from build123d import *

# Parameters (mm, degrees)
SKETCH1_W           = 65.4
SKETCH1_H           = 65.4
BOSS_EXTRUDE1_DEPTH = 1.12
FILLET1_R           = 4
BOSS_EXTRUDE2_START = 10
BOSS_EXTRUDE2_DEPTH = 10
CUT_EXTRUDE1_REACH  = 75.96
SKETCH4_W           = 19.5
SKETCH4_H           = 3.5
CUT_EXTRUDE2_DEPTH  = 2.5
FILLET3_R           = 2
SKETCH5_W           = 1.6
SKETCH5_H           = 49.8
SKETCH5_W_2         = 49.8
SKETCH5_H_2         = 1.6
BOSS_EXTRUDE3_DEPTH = 1
BOSS_EXTRUDE4_DEPTH = 3.8
SKETCH7_R           = 1.55
CUT_EXTRUDE3_DEPTH  = 11.12
SKETCH8_R           = 2.75
CUT_EXTRUDE4_DEPTH  = 4
FILLET4_R           = 1.5
FILLET5_R           = 1.5
CUT_EXTRUDE5_REACH  = 49.807


with BuildPart() as part:
    # Sketch1 → Boss-Extrude1 (new body)
    with BuildSketch(Plane(origin=(0, 0, 0), x_dir=(1, 0, 0), z_dir=(0, 1, 0))):
        Rectangle(SKETCH1_W, SKETCH1_H)
    extrude(amount=BOSS_EXTRUDE1_DEPTH)

    # Fillet1
    fillet1_edges = [part.edges().sort_by_distance(p)[0] for p in [
        (32.7, 0.56, 32.7),
        (-32.7, 0.56, 32.7),
        (-32.7, 0.56, -32.7),
        (32.7, 0.56, -32.7),
    ]]
    fillet(fillet1_edges, radius=FILLET1_R)

    # Sketch2 → Boss-Extrude2 (add)
    with BuildSketch(Plane(origin=(0, 1.12, 0), x_dir=(1, 0, 0), z_dir=(0, 1, 0)).offset(BOSS_EXTRUDE2_START)):
        with BuildLine():
            Line((-32.7, 28.7), (-32.7, -28.7))
            ThreePointArc((-32.7, -28.7), (-31.528427125, -31.528427125), (-28.7, -32.7))
            Line((-28.7, -32.7), (28.7, -32.7))
            ThreePointArc((28.7, -32.7), (31.528427125, -31.528427125), (32.7, -28.7))
            Line((32.7, -28.7), (32.7, 28.7))
            ThreePointArc((32.7, 28.7), (31.528427125, 31.528427125), (28.7, 32.7))
            Line((28.7, 32.7), (-28.7, 32.7))
            ThreePointArc((-28.7, 32.7), (-31.528427125, 31.528427125), (-32.7, 28.7))
        make_face()
        with BuildLine():
            Line((24.9, 28.7), (-24.9, 28.7))
            ThreePointArc((-24.9, 28.7), (-26.012994231, 26.012994231), (-28.7, 24.9))
            Line((-28.7, 24.9), (-28.7, -24.9))
            ThreePointArc((-28.7, -24.9), (-26.012994231, -26.012994231), (-24.9, -28.7))
            Line((-24.9, -28.7), (24.9, -28.7))
            ThreePointArc((24.9, -28.7), (26.012994231, -26.012994231), (28.7, -24.9))
            Line((28.7, -24.9), (28.7, 24.9))
            ThreePointArc((28.7, 24.9), (26.012994231, 26.012994231), (24.9, 28.7))
        make_face(mode=Mode.SUBTRACT)
    extrude(amount=-BOSS_EXTRUDE2_DEPTH)

    # Sketch3 → Cut-Extrude1 (cut, up to next)
    with BuildSketch(Plane(origin=(0, 0, -32.7), x_dir=(-1, 0, 0), z_dir=(0, 0, -1)), mode=Mode.PRIVATE) as cut_extrude1_sk1:
        with BuildLine():
            Line((-3, 6.5), (3, 6.5))
            ThreePointArc((3, 6.5), (5, 4.5), (3, 2.5))
            Line((3, 2.5), (-3, 2.5))
            ThreePointArc((-3, 2.5), (-5, 4.5), (-3, 6.5))
        make_face()
    cut_extrude1_tool1 = extrude(cut_extrude1_sk1.sketch, amount=-CUT_EXTRUDE1_REACH, mode=Mode.PRIVATE) & part.part
    add(cut_extrude1_tool1.solids().sort_by_distance((0, 4.5, -32.7))[0], mode=Mode.SUBTRACT)

    # Sketch4 → Cut-Extrude2 (cut)
    with BuildSketch(Plane.XY.offset(-28.7)):
        with Locations((0, 2.87)):
            Rectangle(SKETCH4_W, SKETCH4_H)
    extrude(amount=-CUT_EXTRUDE2_DEPTH, mode=Mode.SUBTRACT)

    # Fillet3
    # the kernel refuses this fillet: 2 mm, written as the material it takes off along each edge
    with BuildSketch(Plane(origin=(-0.003603246, 4.62, -28.7), x_dir=(0, 1, 0), z_dir=(1, 0, 0)), Plane(origin=(-9.75, 4.62, -28.7), x_dir=(0, 1, 0), z_dir=(1, 0, 0))) as fillet3_piece_1:
        with BuildLine():
            CenterArc((FILLET3_R, -FILLET3_R), FILLET3_R, 90, 90)
            Line((0, -FILLET3_R), (0, 0))
            Line((0, 0), (FILLET3_R, 0))
        make_face()
    extrude(amount=9.753603246, mode=Mode.SUBTRACT)

    # Sketch5 → Boss-Extrude3 (add)
    with BuildSketch(Plane(origin=(0, 11.12, 0), x_dir=(1, 0, 0), z_dir=(0, 1, 0))):
        with Locations((-29.5, 0)):
            Rectangle(SKETCH5_W, SKETCH5_H)
        with Locations((0, -29.5)):
            Rectangle(SKETCH5_W_2, SKETCH5_H_2)
        with Locations((29.5, 0)):
            Rectangle(SKETCH5_W, SKETCH5_H)
        with Locations((0, 29.5)):
            Rectangle(SKETCH5_W_2, SKETCH5_H_2)
    extrude(amount=BOSS_EXTRUDE3_DEPTH)

    # Sketch6 → Boss-Extrude4 (add)
    with BuildSketch(Plane(origin=(0, 1.12, 0), x_dir=(1, 0, 0), z_dir=(0, 1, 0))):
        Polygon((-9.5, -4.3), (9.5, -4.3), (9.5, 1.7), (11.5, 1.7), (11.5, -6.3), (-11.5, -6.3), (-11.5, 1.7), (-9.5, 1.7), align=None)
    extrude(amount=BOSS_EXTRUDE4_DEPTH)

    # Sketch7 → Cut-Extrude3 (cut)
    with BuildSketch(Plane(origin=(0, 11.12, 0), x_dir=(1, 0, 0), z_dir=(0, 1, 0))):
        with Locations(Location((-28.9, 28.9, 0), (0, 0, 270))):
            Circle(SKETCH7_R)
        with Locations(Location((28.9, 28.9, 0), (0, 0, 270))):
            Circle(SKETCH7_R)
        with Locations(Location((28.9, -28.9, 0), (0, 0, 270))):
            Circle(SKETCH7_R)
        with Locations(Location((-28.9, -28.9, 0), (0, 0, 270))):
            Circle(SKETCH7_R)
    extrude(amount=-CUT_EXTRUDE3_DEPTH, mode=Mode.SUBTRACT)

    # Sketch8 → Cut-Extrude4 (cut)
    with BuildSketch(Plane.XZ):
        with Locations(Location((-28.9, 28.9, 0), (0, 0, 270))):
            Circle(SKETCH8_R)
        with Locations(Location((28.9, 28.9, 0), (0, 0, 270))):
            Circle(SKETCH8_R)
        with Locations(Location((28.9, -28.9, 0), (0, 0, 270))):
            Circle(SKETCH8_R)
        with Locations(Location((-28.9, -28.9, 0), (0, 0, 270))):
            Circle(SKETCH8_R)
    extrude(amount=-CUT_EXTRUDE4_DEPTH, mode=Mode.SUBTRACT)

    # Fillet4
    fillet4_edges = [part.edges().sort_by_distance(p)[0] for p in [
        (-11.5, 1.12, 2.3),
        (0, 1.12, 6.3),
        (11.5, 1.12, 2.3),
    ]]
    fillet(fillet4_edges, radius=FILLET4_R)

    # Fillet5
    fillet5_edges = [part.edges().sort_by_distance(p)[0] for p in [
        (-17.325, 1.12, -28.7),
        (26.012994231, 1.12, -26.012994231),
        (17.325, 1.12, -28.7),
        (-26.012994231, 1.12, -26.012994231),
        (-28.7, 1.12, 0),
        (-26.012994231, 1.12, 26.012994231),
        (0, 1.12, 28.7),
        (26.012994231, 1.12, 26.012994231),
        (28.7, 1.12, 0),
    ]]
    fillet(fillet5_edges, radius=FILLET5_R)

    # Sketch9 → Cut-Extrude5 (cut, up to next)
    with BuildSketch(Plane.XZ, mode=Mode.PRIVATE) as cut_extrude5_sk1:
        with BuildLine():
            Line((6.45, -23), (6.45, -20))
            ThreePointArc((6.45, -20), (7.7, -18.75), (8.95, -20))
            Line((8.95, -20), (8.95, -23))
            ThreePointArc((8.95, -23), (7.7, -24.25), (6.45, -23))
        make_face()
    cut_extrude5_tool1 = extrude(cut_extrude5_sk1.sketch, amount=-CUT_EXTRUDE5_REACH, mode=Mode.PRIVATE) & part.part
    add(cut_extrude5_tool1.solids().sort_by_distance((7.7, 0, -21.5))[0], mode=Mode.SUBTRACT)


solid = part.part
Design review of the part built by this model. Coordinates are the model's own, in mm. A direction names the side the tool comes from. Round coordinates to 2 decimals unless told otherwise and drop trailing zeros. Loops run counter-clockwise (first coordinate to the right, second up) from the corner with the lowest first, then second, coordinate; pieces in that order, holes last. Notation, with made-up numbers: M 37.5,-39 L 95.5,-39 A21 cw 95.5,-1 Z; hole C 19.25,37.25 d4. An arc over 180 degrees is marked long. Answer as a JSON object with one key per item and string values.
Item 1: Wall thickness on L1, parallel to X at y = 10.5, z = -29; L2, parallel to Z at x = -18.5, y = 8.25: over which ranges is each line inside the solid? List them lowest first. Write a range as from..to.
Answer sheet:
{"L1": "x = -32.69..-30.45, -27.35..27.35, 30.45..32.69", "L2": "z = -32.7..-28.7, 28.7..32.7"}
Item 2: We need section A-A on x = 7.7. Give the boundary of the cut face in (y, z), and give its area (3 significant figures).
Answer sheet:
{"outline": "M 0,-32.7 L 11.12,-32.7 L 11.12,-30.3 L 12.12,-30.3 L 12.12,-28.7 L 6.62,-28.7 A2 ccw 4.62,-30.7 L 4.62,-31.2 L 1.12,-31.2 L 1.12,-24.25 L 0,-24.25 Z; M 0,-18.75 L 1.12,-18.75 L 1.12,4.3 L 4.92,4.3 L 4.92,6.3 L 2.62,6.3 A1.5 cw 1.12,7.8 L 1.12,27.2 A1.5 cw 2.62,28.7 L 12.12,28.7 L 12.12,30.3 L 11.12,30.3 L 11.12,32.7 L 0,32.7 Z", "area": "149 mm^2"}
Item 3: We need section B-B on z = -7.5. Give the boundary of the cut face in (x, y), and give its area (3 significant figures).
Answer sheet:
{"outline": "M -32.7,0 L 32.7,0 L 32.7,11.12 L 30.3,11.12 L 30.3,12.12 L 28.7,12.12 L 28.7,2.62 A1.5 cw 27.2,1.12 L -27.2,1.12 A1.5 cw -28.7,2.62 L -28.7,12.12 L -30.3,12.12 L -30.3,11.12 L -32.7,11.12 Z", "area": "157 mm^2"}
Item 4: Clearance check with flat-ended pins moving along their axes: P1, Ø0.8, axis at y = 12, z = -9.5, coming from the +X side; P2, Ø1.1, axis at y = 11.5, z = 29.5, coming from the +X side; P3, Ø5, axis at x = -28.9, z = -28.9, coming from the -Y side. State where each tip first meets the part, or that it passes through.
Answer sheet:
{"P1": "stops at x = 30.3", "P2": "stops at x = 32.68", "P3": "stops at y = 4"}
Item 5: The part is to be moulded in two halves that separate along Z. For faces 4 (the flat face through (0, 12.12, -30)), 5 (the cylindrical face through (17.2, 1.5, -28.2)), say which applies: pulls with the +Z half, pulls with the -Z half, needs draft (parallel to the pull), parting line crosses it, or undercut.
Answer sheet:
{"face 4": "needs draft", "face 5": "undercut"}
Item 6: We need section C-C on x = -8.5. Give the boundary of the cut face in (y, z), and give its area (3 significant figures).
Answer sheet:
{"outline": "M 0,-32.7 L 11.12,-32.7 L 11.12,-30.3 L 12.12,-30.3 L 12.12,-28.7 L 6.62,-28.7 A2 ccw 4.62,-30.7 L 4.62,-31.2 L 1.12,-31.2 L 1.12,4.3 L 4.92,4.3 L 4.92,6.3 L 2.62,6.3 A1.5 cw 1.12,7.8 L 1.12,27.2 A1.5 cw 2.62,28.7 L 12.12,28.7 L 12.12,30.3 L 11.12,30.3 L 11.12,32.7 L 0,32.7 Z", "area": "155 mm^2"}
Item 7: Machinability: for faces 1 (the flat face through (29, 4, -31)), 2 (the flat face through (9.75, 3, -30)), 3 (the cylindrical face through (12, 1.5, 3.1)), which of the approach directions +Z, -Z, +X, -X, +Y, -Y give a long, thin tool a straight path to every point of the face, cutting with its end or side? Answer none if there is none.
Answer sheet:
{"face 1": "-Y", "face 2": "none", "face 3": "+Y"}
